Work out the finished part from the listing and answer in its coordinate system (mm). A direction names the side the tool comes from. Give positions to 0.01 mm unless a question says otherwise; leave off trailing zeros. Write each loop counter-clockwise with the first axis right and the second up, starting at its lowest first coordinate (ties: lowest second). Pieces come first, ordered by that corner, then holes.
1) Straight lines are drawn through the part: probe 1 along Z at (x, y) = (8.75, -3.75); probe 2 along Y at (x, z) = (0.5, 2.25); probe 3 along Z at (x, y) = (10, 4.75). For each, find the intervals that lie inside material, in ascending order.
2) A tool of negligible diameter and unlimited length cuts with its end or side. For faces 1 (the face through (0.617, -6.424, 4.656)), 2 (the face through (1, -4.5, 2)), 3 (the face through (0, -6.5, 1)), from which of +Z, -Z, +X, -X, +Y, -Y can it reach the whole face along a straight path? Write none if from no direction.
3) Find section B-B (y = -4.25). Determine the outline of the cut face in (x, z), plus the area to 3 significant figures.
4) Find section C-C (z = 4.75). Determine the outline of the cut face in (x, y), plus the area to 3 significant figures.
5) Find section A-A (x = 3.25). Determine the outline of the cut face in (y, z), plus the area to 3 significant figures.
6) Given pin 1 Ø3 at (x, y) = (-6, 0) entering from +Z; pin 2 Ø0.9 at (x, z) = (1, 2) entering from +Y; pin 3 Ø3 at (x, z) = (-4, 4) entering from -Y; pin 4 Ø1.5 at (y, z) = (-4.5, 2) entering from -X, each flat-ended and moving along its own axis, determine where each tip first touches the part or whether it passes through.
```python
from build123d import *

# Parameters (mm, degrees)
AUFSATZ_LINEAR_AUSTRAGEN1_DEPTH = 1.6
SKIZZE1_3_R                     = 1.0000000000000002
AUFSATZ_LINEAR_AUSTRAGEN2_DEPTH = 6
AUFSATZ_LINEAR_AUSTRAGEN3_DEPTH = 3.35
FASE1_SIZE                      = 1
FASE2_SIZE                      = 1.6
FASE2_SIZE_2                    = 0.4
FASE3_SIZE                      = 0.4
FASE3_SIZE_2                    = 1.6
FASE4_SIZE                      = 2.771281292
FASE4_SIZE_2                    = 1.6


# Some blends are built 0.0001 mm under size
with BuildPart() as part:
    # Skizze1 → Aufsatz-Linear austragen1 (new body)
    with BuildSketch(Plane.XY):
        Polygon((-13, 6.500000000000001), (13, 6.500000000000001), (13.000000000000004, -6.499999999999999), (-12.999999999999998, -6.499999999999999), align=None)
    extrude(amount=AUFSATZ_LINEAR_AUSTRAGEN1_DEPTH)

    # Skizze1<3> → Aufsatz-Linear austragen2 (add)
    with BuildSketch(Plane.XY):
        with Locations(Location((1.0000000000000009, -5.499999999999999, 0), (0, 0, 270))):
            Circle(SKIZZE1_3_R)
    extrude(amount=AUFSATZ_LINEAR_AUSTRAGEN2_DEPTH)

    # Skizze1<4> → Aufsatz-Linear austragen3 (add)
    with BuildSketch(Plane.XY):
        with BuildLine():
            ThreePointArc((-0.732050807568877, -4.499999999999999), (-0.9999999999999996, -5.4999999999999885), (-0.7320508075688883, -6.49999999999998))
            Line((-0.7320508075688945, -6.499999999999999), (1.000000000000023, -6.499999999999999))
            ThreePointArc((1.0000000000000238, -6.499999999999999), (6.7e-16, -5.499999999999999), (1.000000000000023, -4.499999999999999))
            Line((1.000000000000023, -4.499999999999999), (-0.732050807568877, -4.499999999999999))
        make_face()
        with BuildLine():
            Line((1.000000000000023, -6.499999999999999), (2.7320508075688927, -6.499999999999999))
            ThreePointArc((2.732050807568887, -6.499999999999985), (2.93185165257814, -6.0176380902050335), (3.0000000000000013, -5.5))
            ThreePointArc((3.0000000000000013, -5.499999999999999), (2.931851652578138, -4.982361909794958), (2.7320508075688785, -4.499999999999999))
            Line((2.7320508075688785, -4.499999999999999), (1.000000000000023, -4.499999999999999))
            ThreePointArc((1.000000000000023, -4.499999999999999), (1.7071067811865563, -4.792893218813459), (2.000000000000001, -5.499999999999999))
            ThreePointArc((2.000000000000001, -5.499999999999999), (1.7071067811865566, -6.207106781186539), (1.0000000000000238, -6.499999999999999))
        make_face()
    extrude(amount=AUFSATZ_LINEAR_AUSTRAGEN3_DEPTH)

    # Fase1
    fase1_edges = [part.edges().sort_by_distance(p)[0] for p in [
        (3.0000000000000018, -5.499999999999993, 3.35),
        (-1, -5.499999999999988, 3.35),
    ]]
    chamfer(fase1_edges, length=FASE1_SIZE - 0.0001)  # a hair under: the kernel refuses the full size

    # Fase2
    # the kernel refuses this chamfer: 1.6, 0.4 mm, written as the material it takes off along each edge
    with BuildSketch(Plane(origin=(12.999999999999998, 10.655403999635418, 0), x_dir=(0.009338610640317949, 0, 0.9999563942249226), z_dir=(2.7e-16, -1, 0))) as fase2_piece_1:
        Polygon((FASE2_SIZE * 0.999956394225, FASE2_SIZE * 0.00933861064032), (-FASE2_SIZE_2 * 0.00933861064032, FASE2_SIZE_2 * 0.999956394225), (0, 0), align=None)
    extrude(amount=21.310807999270835, mode=Mode.SUBTRACT)

    # Fase3
    # the kernel refuses this chamfer: 1.6, 0.4 mm, written as the material it takes off along each edge
    with BuildSketch(Plane(origin=(-12.999999999999998, -10.655403999635418, 0), x_dir=(0.9890197255468893, 0, -0.1477835663365709), z_dir=(-1.4e-16, 1, 0))) as fase3_piece_1:
        Polygon((FASE3_SIZE * 0.989019725547, -FASE3_SIZE * 0.147783566337), (-FASE3_SIZE_2 * 0.147783566337, -FASE3_SIZE_2 * 0.989019725547), (0, 0), align=None)
    extrude(amount=21.310807999270835, mode=Mode.SUBTRACT)

    # Fase4
    # the kernel refuses this chamfer: 2.771281292, 1.6 mm, written as the material it takes off along each edge
    with BuildSketch(Plane(origin=(-20.169542352935284, 6.500000000000001, 1.6), x_dir=(0, -0.999813220622208, 0.01932676561270061), z_dir=(1, 0, 0))) as fase4_piece_1:
        Polygon((FASE4_SIZE * 0.999813220662, FASE4_SIZE * 0.0193267656135), (-FASE4_SIZE_2 * 0.0193267656127, FASE4_SIZE_2 * 0.999813220622), (0, 0), align=None)
    extrude(amount=40.33908470587056, mode=Mode.SUBTRACT)


solid = part.part
```
Results:
1. probe 1: z = 0 to 1.6
1. probe 2: y = -6.5 to -4.5
1. probe 3: z = 0 to 1.01
2. face 1: +Z
2. face 2: +Z, +X, -X, +Y
2. face 3: +Z, -Z, +X, -X, -Y
3. outline: (-13, 1.6) - (-12.6, 0) - (12.6, 0) - (13, 1.6) - close
3. area: 41.0 mm2
4. outline: circle Ø2 at (1, -5.5)
4. area: 3.14 mm2
5. outline: (-6.5, 0) - (6.5, 0) - (3.73, 1.6) - (-6.5, 1.6) - close
5. area: 18.6 mm2
6. pin 1: stops at z = 1.6
6. pin 2: stops at y = 3.82
6. pin 3: passes through
6. pin 4: stops at x = -13
